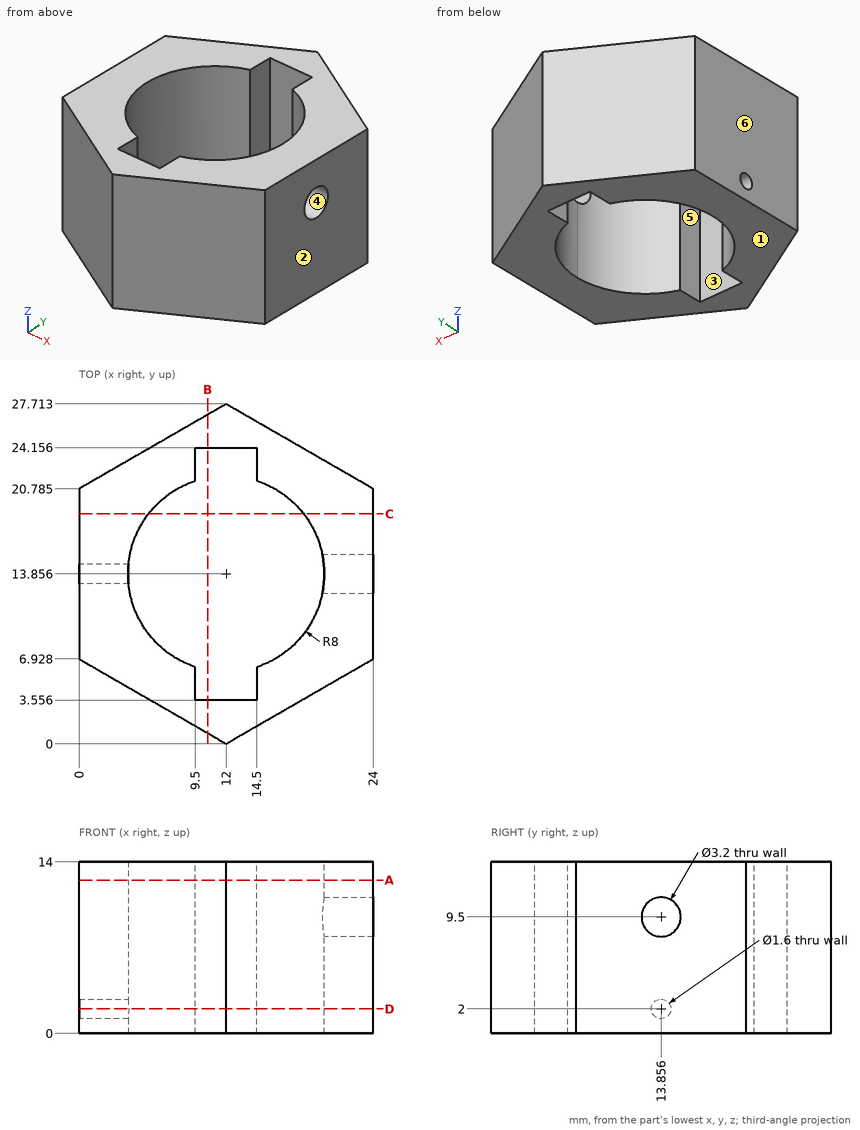
Could you check a few things on this drawing? It's one solid part, dimensions in mm from its lowest x, y, z. A direction names the side the tool comes from. Coordinates: 2 decimals unless noted, no trailing zeros. Loops run counter-clockwise (first coordinate to the right, second up) from the corner with the lowest first, then second, coordinate; pieces in that order, holes last. Notation, with made-up numbers: (17, 69.25) - (23, 69.25) arc R16 ccw to (23, 79.25) - close; hole circle Ø10 at (-21.5, 35). An arc over 180 degrees is marked (long way). Return JSON: item names as keys, results as strings. Group by question number.
Item 1: If we section it at D-D on z = 2: Write out the boundary of the cut face in (x, y) (1 decimal), and give its area (3 significant figures).
Item 2: If we section it at B-B on x = 10.5: Write out the boundary of the cut face in (y, z).
Item 3: I need wall thicknesses on line 1 (Y direction, x = 13.25, z = 3.25) (1 decimal); line 2 (Y direction, x = 8.75, z = 3.75) (1 decimal); line 3 (X direction, y = 10.75, z = 1). Which ranges of each line are inside material? Lowest first, please. Write a range as from..to.
Item 4: On a 3-axis mill with a long thin cutter (end or side, diameter ignored), from which of +Z, -Z, +X, -X, +Y, -Y can I reach the whole of each face in a straight line? I mean the marked faces 4, 5 and 6. Say none if no direction works.
Item 5: We'd pull the mould along X, two halves only. Please class the marked faces 1, 2 and 3: +X half, -X half, draft (parallel to the pull), parting line (faces both ways), or undercut.
Item 6: Will these pins go through, and if not, where does the flat tip stop? P1, Ø1.5, axis at x = 11.5, z = 10, coming from the -Y side; P2, Ø8, axis at x = 11, y = 17.5, coming from the +Z side; P3, Ø4, axis at x = 11, z = 8.5, coming from the +Y side; P4, Ø3.5, axis at y = 13.86, z = 9.5, coming from the +X side.
Item 7: If we section it at A-A on z = 12.5: Write out the boundary of the cut face in (x, y) (1 decimal).
Item 8: If we section it at C-C on y = 18.75: Write out the boundary of the cut face in (x, z).
Calculated:
{
 "1": {"outline": "(0, 6.9) - (12, 0) - (24, 6.9) - (24, 20.8) - (12, 27.7) - (0, 20.8) - (0, 14.7) - (4, 14.7) arc R8 cw to (9.5, 21.5) - (9.5, 24.2) - (14.5, 24.2) - (14.5, 21.5) arc R8 cw to (14.5, 6.3) - (14.5, 3.6) - (9.5, 3.6) - (9.5, 6.3) arc R8 cw to (4, 13.1) - (0, 13.1) - close", "area": "267 mm^2"},
 "2": {"outline": "(0.87, 0) - (3.56, 0) - (3.56, 14) - (0.87, 14) - close; (24.16, 0) - (26.85, 0) - (26.85, 14) - (24.16, 14) - close"},
 "3": {"line 1": "y = 0.7..3.6, 24.2..27", "line 2": "y = 1.9..6.5, 21.2..25.8", "line 3": "x = 0..4.63, 19.37..24"},
 "4": {"face 4": "+X", "face 5": "+Z, -Z", "face 6": "+Z, -Z, -X, +Y, -Y"},
 "5": {"face 1": "draft", "face 2": "+X half", "face 3": "undercut"},
 "6": {"P1": "stops at y = 0", "P2": "passes through", "P3": "stops at y = 27.71", "P4": "stops at x = 24"},
 "7": {"outline": "(0, 6.9) - (12, 0) - (24, 6.9) - (24, 20.8) - (12, 27.7) - (0, 20.8) - close; hole (9.5, 3.6) - (14.5, 3.6) - (14.5, 6.3) arc R8 ccw to (14.5, 21.5) - (14.5, 24.2) - (9.5, 24.2) - (9.5, 21.5) arc R8 ccw to (9.5, 6.3) - close"},
 "8": {"outline": "(0, 0) - (5.67, 0) - (5.67, 14) - (0, 14) - close; (18.33, 0) - (24, 0) - (24, 14) - (18.33, 14) - close"}
}
